Model file for the job. Use its own axes, mm. Face numbers are marked on the shaded views. A direction names the side the tool comes from. Round coordinates to 2 decimals unless told otherwise and drop trailing zeros. Order: outer loops, then holes, each group sorted by start corner. A loop starts at its lowest first (then second) coordinate and runs counter-clockwise, first axis right, second up. Notation, with made-up numbers: (68.25, 38.25) - (94.25, 38.25) arc R27 ccw to (94.25, 63.25) - close; hole circle Ø10 at (65, -9.5). An arc over 180 degrees is marked (long way). Use one line per item in the form item = value.
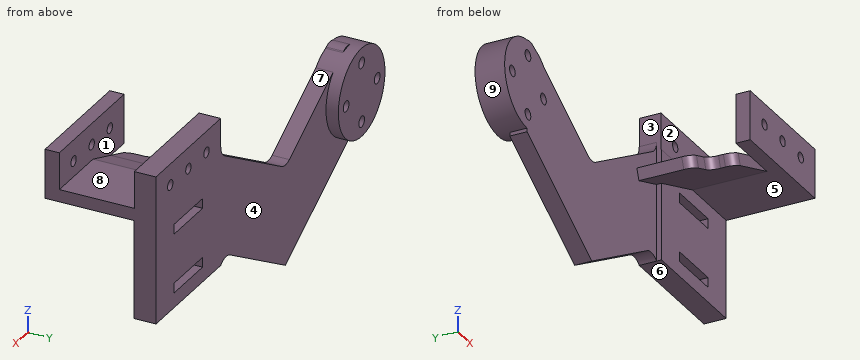
from build123d import *

# Parameters (mm, degrees)
SKETCH_1_W               = 25
SKETCH_1_H               = 10
EXTRUDE_1_DEPTH          = 22.5
SKETCH_2_W               = 25
SKETCH_2_H               = 15.2
CUT_EXTRUDE_1_DEPTH      = 7.5
CUT_EXTRUDE_2_DEPTH      = 36.089172119
CUT_EXTRUDE_2_DEPTH_BACK = 36.089172119
SKETCH_4_R               = 1.03
SKETCH_5_W               = 25
SKETCH_5_H               = 4.5
EXTRUDE_2_DEPTH          = 20
SKETCH_6_W               = 11
SKETCH_6_H               = 2
CUT_EXTRUDE_3_DEPTH      = 4.5
EXTRUDE_3_DEPTH          = 3.5
SKETCH_16_R              = 9
EXTRUDE_4_DEPTH          = 6
CUT_EXTRUDE_4_REACH      = 71.426
SKETCH_17_R              = 1.1
CUT_EXTRUDE_5_REACH      = 73.302
SKETCH_19_W              = 12
SKETCH_19_H              = 15.1
FILLET_7_R               = 3
EXTRUDE_6_REACH          = 72.338
CUT_EXTRUDE_6_REACH      = 72.847
SKETCH_22_W              = 7
SKETCH_22_H              = 5
FILLET_8_R               = 2


with BuildPart() as part:
    # 草图1 → 凸台-拉伸1 (new body)
    with BuildSketch(Plane(origin=(0, 0, 0), x_dir=(1, 0, 0), z_dir=(0, 1, 0))):
        with Locations((12.5, -5)):
            Rectangle(SKETCH_1_W, SKETCH_1_H)
    extrude(amount=EXTRUDE_1_DEPTH)

    # 草图2 → 切除-拉伸1 (cut)
    with BuildSketch(Plane.XY.offset(10)):
        with Locations((12.5, 10.5)):
            Rectangle(SKETCH_2_W, SKETCH_2_H)
    extrude(amount=-CUT_EXTRUDE_1_DEPTH, mode=Mode.SUBTRACT)

    # 草图4 → 切除-拉伸2 (cut, two sides: drawn at the far end of the back side and taken through both)
    with BuildSketch(Plane(origin=(0, 22.5, 0), x_dir=(1, 0, 0), z_dir=(0, 1, 0)).offset(-CUT_EXTRUDE_2_DEPTH_BACK)):
        with Locations(Location((12.5, -5.7, 0), (0, 0, 270))):
            Circle(SKETCH_4_R)
        with Locations(Location((19.5, -5.7, 0), (0, 0, 270))):
            Circle(SKETCH_4_R)
        with Locations(Location((5.5, -5.7, 0), (0, 0, 270))):
            Circle(SKETCH_4_R)
    extrude(amount=CUT_EXTRUDE_2_DEPTH + CUT_EXTRUDE_2_DEPTH_BACK, mode=Mode.SUBTRACT)

    # 草图5 → 凸台-拉伸2 (add)
    with BuildSketch(Plane(origin=(0, 0, 0), x_dir=(-1, 0, 0), z_dir=(0, 0, -1))):
        with Locations((-12.5, 20.25)):
            Rectangle(SKETCH_5_W, SKETCH_5_H)
    extrude(amount=EXTRUDE_2_DEPTH)

    # 草图6 → 切除-拉伸3 (cut)
    with BuildSketch(Plane(origin=(0, 22.5, 0), x_dir=(1, 0, 0), z_dir=(0, 1, 0))):
        with Locations((12.5, 16)):
            Rectangle(SKETCH_6_W, SKETCH_6_H)
        with Locations((12.5, 4)):
            Rectangle(SKETCH_6_W, SKETCH_6_H)
    extrude(amount=-CUT_EXTRUDE_3_DEPTH, mode=Mode.SUBTRACT)

    # 草图15 → 凸台-拉伸3 (add)
    with BuildSketch(Plane(origin=(0, 22.5, 0), x_dir=(1, 0, 0), z_dir=(0, 1, 0))):
        Polygon((0, 17.5), (0, -2.5), (-25, 11.93375673), (-50, -2.5), (-50, 17.5), (-24.967235844, 31.914840335), align=None)
    extrude(amount=-EXTRUDE_3_DEPTH)

    # 草图16 → 凸台-拉伸4 (add)
    with BuildSketch(Plane.XZ.offset(-19)):
        with Locations(Location((-49.655444566, -7.782050808, 0), (0, 0, 267.805955804))):
            Circle(SKETCH_16_R)
    extrude(amount=-EXTRUDE_4_DEPTH)

    # 草图17 → 切除-拉伸4 (cut, up to next)
    with BuildSketch(Plane.XZ.offset(-19), mode=Mode.PRIVATE) as cut_extrude_4_sk1:
        with Locations(Location((-55.655444566, -7.782050808, 0), (0, 0, 90))):
            Circle(SKETCH_17_R)
    cut_extrude_4_tool1 = extrude(cut_extrude_4_sk1.sketch, amount=-CUT_EXTRUDE_4_REACH, mode=Mode.PRIVATE) & part.part
    # 草图17 → 切除-拉伸4 (cut, up to next)
    with BuildSketch(Plane.XZ.offset(-19), mode=Mode.PRIVATE) as cut_extrude_4_sk2:
        with Locations(Location((-43.655444566, -7.782050808, 0), (0, 0, 90))):
            Circle(SKETCH_17_R)
    cut_extrude_4_tool2 = extrude(cut_extrude_4_sk2.sketch, amount=-CUT_EXTRUDE_4_REACH, mode=Mode.PRIVATE) & part.part
    # 草图17 → 切除-拉伸4 (cut, up to next)
    with BuildSketch(Plane.XZ.offset(-19), mode=Mode.PRIVATE) as cut_extrude_4_sk3:
        with Locations(Location((-49.655444566, -1.782050808, 0), (0, 0, 90))):
            Circle(SKETCH_17_R)
    cut_extrude_4_tool3 = extrude(cut_extrude_4_sk3.sketch, amount=-CUT_EXTRUDE_4_REACH, mode=Mode.PRIVATE) & part.part
    # 草图17 → 切除-拉伸4 (cut, up to next)
    with BuildSketch(Plane.XZ.offset(-19), mode=Mode.PRIVATE) as cut_extrude_4_sk4:
        with Locations(Location((-49.655444566, -13.782050808, 0), (0, 0, 90))):
            Circle(SKETCH_17_R)
    cut_extrude_4_tool4 = extrude(cut_extrude_4_sk4.sketch, amount=-CUT_EXTRUDE_4_REACH, mode=Mode.PRIVATE) & part.part
    add(cut_extrude_4_tool1.solids().sort_by_distance((-55.655445, 19, -7.782051))[0], mode=Mode.SUBTRACT)
    add(cut_extrude_4_tool2.solids().sort_by_distance((-43.655445, 19, -7.782051))[0], mode=Mode.SUBTRACT)
    add(cut_extrude_4_tool3.solids().sort_by_distance((-49.655445, 19, -1.782051))[0], mode=Mode.SUBTRACT)
    add(cut_extrude_4_tool4.solids().sort_by_distance((-49.655445, 19, -13.782051))[0], mode=Mode.SUBTRACT)

    # 草图19 → 切除-拉伸5 (cut, up to next)
    with BuildSketch(Plane(origin=(0, 0, 0), x_dir=(-1, 0, 0), z_dir=(0, 0, -1)), mode=Mode.PRIVATE) as cut_extrude_5_sk1:
        with Locations((-6, 10.45)):
            Rectangle(SKETCH_19_W, SKETCH_19_H)
    cut_extrude_5_tool1 = extrude(cut_extrude_5_sk1.sketch, amount=-CUT_EXTRUDE_5_REACH, mode=Mode.PRIVATE) & part.part
    add(cut_extrude_5_tool1.solids().sort_by_distance((6, 10.45, 0))[0], mode=Mode.SUBTRACT)

    # 圆角7
    # the kernel refuses this fillet: 3 mm, written as the material it adds along each edge
    with BuildSketch(Plane(origin=(0, 22.5, -17.5), x_dir=(-0.866025403784437, 0, -0.5000000000000027), z_dir=(0, -1, 0))) as fillet_7_piece_1:
        with BuildLine():
            CenterArc((4.131472029, 3), FILLET_7_R, 196.159495152, 73.840504848)
            Line((1.25, 2.165063509), (0, 0))
            Line((0, 0), (4.131472029, 0))
        make_face()
    extrude(amount=3.5)
    with BuildSketch(Plane(origin=(0, 22.5, 2.5), x_dir=(-0.8660254037844379, 0, -0.5000000000000012), z_dir=(0, -1, 0))) as fillet_7_piece_2:
        with BuildLine():
            CenterArc((FILLET_7_R * 0.57735026919, -FILLET_7_R), FILLET_7_R, 90, 60)
            Line((-FILLET_7_R * 0.288675134595, -FILLET_7_R * 0.5), (0, 0))
            Line((0, 0), (FILLET_7_R * 0.57735026919, 0))
        make_face()
    extrude(amount=3.5)
    with BuildSketch(Plane(origin=(-25, 22.5, -11.93375673), x_dir=(0.8660254037844384, 0, 0.5000000000000003), z_dir=(0, -1, 0))) as fillet_7_piece_3:
        with BuildLine():
            CenterArc((FILLET_7_R * 0.57735026919, FILLET_7_R), FILLET_7_R, 210, 60)
            Line((-FILLET_7_R * 0.288675134595, FILLET_7_R * 0.5), (0, 0))
            Line((0, 0), (FILLET_7_R * 0.57735026919, 0))
        make_face()
    extrude(amount=3.5)
    # the kernel refuses this fillet: 3 mm, written as the material it takes off along each edge
    with BuildSketch(Plane(origin=(-50, 29.947415965, 2.5), x_dir=(0, 0, -1), z_dir=(0, -1, 0))) as fillet_7_2_piece_1:
        with BuildLine():
            CenterArc((4.087559404, 1.079860567), FILLET_7_R, 150, 51.097341704)
            Line((1.489483193, 2.579860567), (0, 0))
            Line((0, 0), (1.288648696, 0))
        make_face()
    extrude(amount=18.394831929, mode=Mode.SUBTRACT)

    # 凸台-拉伸6: up to this face of the body (flat: up to its plane)
    extrude_6_end = Plane(part.part.faces().sort_by_distance((-27.69980279, 19, -14.058564272))[0])
    # 草图21 → 凸台-拉伸6 (add, up to the picked face)
    with BuildSketch(Plane(origin=(0, 2.9, 0), x_dir=(1, 0, 0), z_dir=(0, 1, 0)), mode=Mode.PRIVATE) as extrude_6_sk1:
        Polygon((5.131306451, 0), (12, 0), (-6.793852416, 6.840402867), (-7.597336928, 4.632847313), align=None)
    extrude_6_tool1 = split(extrude(extrude_6_sk1.sketch, amount=EXTRUDE_6_REACH, mode=Mode.PRIVATE), bisect_by=extrude_6_end, keep=Keep.BOTH, mode=Mode.PRIVATE)
    # 草图21 → 凸台-拉伸6 (add, up to the picked face)
    with BuildSketch(Plane(origin=(0, 2.9, 0), x_dir=(1, 0, 0), z_dir=(0, 1, 0)), mode=Mode.PRIVATE) as extrude_6_sk2:
        Polygon((5.131306451, 0), (12, -2.5), (12, 0), align=None)
    extrude_6_tool2 = split(extrude(extrude_6_sk2.sketch, amount=EXTRUDE_6_REACH, mode=Mode.PRIVATE), bisect_by=extrude_6_end, keep=Keep.BOTH, mode=Mode.PRIVATE)
    add(extrude_6_tool1.solids().sort_by(Axis((0.808046, 2.9, -2.903709), (0, 1, 0)))[0])
    add(extrude_6_tool2.solids().sort_by(Axis((9.710435, 2.9, 0.833333), (0, 1, 0)))[0])

    # 草图22 → 切除-拉伸6 (cut, up to next)
    with BuildSketch(Plane(origin=(1.403733341, 0, -3.856725658), x_dir=(-0.9396926207859082, 0, -0.3420201433256691), z_dir=(0.3420201433256691, 0, -0.9396926207859082)), mode=Mode.PRIVATE) as cut_extrude_6_sk1:
        with Locations((5.223688551, 5.4)):
            Rectangle(SKETCH_22_W, SKETCH_22_H)
    cut_extrude_6_tool1 = extrude(cut_extrude_6_sk1.sketch, amount=-CUT_EXTRUDE_6_REACH, mode=Mode.PRIVATE) & part.part
    add(cut_extrude_6_tool1.solids().sort_by_distance((-3.504928, 5.4, -5.643332))[0], mode=Mode.SUBTRACT)

    # 圆角8
    fillet_8_edges = [part.edges().sort_by_distance(p)[0] for p in [
        (-7.195594672, 7.9, -5.73662509),
        (-0.617746326, 2.9, -3.342484086),
        (-0.617746326, 7.9, -3.342484086),
    ]]
    fillet(fillet_8_edges, radius=FILLET_8_R)


solid = part.part
(1) Slice it at C-C on x = 2.5. Give the cut face in (y, z).
Report:
outline = (0, 0) - (2.9, 0) - (2.9, 10) - (0, 10) - close; (2.9, -3.46) - (18, -3.46) - (18, -20) - (22.5, -20) - (22.5, 10) - (18.1, 10) - (18.1, 2.5) - (18, 2.5) - (18, -0.96) - (2.9, -0.96) - close
(2) Tool access for the marked faces 5, 6, 7, 8 and 9: list every direction of +Z, -Z, +X, -X, +Y, -Y with a clear straight run to the whole face (end or side of a thin tool).
Report:
face_5 = -Z, +X, -Y
face_6 = -Z, +X, +Y, -Y
face_7 = +Z, +Y, -Y
face_8 = +Z, +X, -X
face_9 = +Y
(3) Slice it at D-D on y = 21.25. Count the separate pieces of the cut face and the enclosed holes in it, then the cut area to 3 significant figures.
Report:
separate_pieces = 1
enclosed_holes = 9
area = 1,800 mm2
(4) Pull direction Y, two halves, no side cores. Call the marked faces 1, 2, 3 and 4: released by +Y, released by -Y, zero draft, split by the parting line, or undercut.
Report:
face_1 = undercut
face_2 = undercut
face_3 = zero draft
face_4 = released by +Y
(5) Slice it at B-B on y = 16.75. Give the cut face in (x, z), then the cut area to 3 significant figures.
Report:
outline = (-7.6, -4.63) - (-6.79, -6.84) - (12, 0) - (25, 0) - (25, 2.5) - (12, 2.5) - close
area = 80.5 mm2
(6) Pin check, flat tips, straight feed: pin 1 (2.5 mm diameter, centred on x = -3.5, z = -4.5, fed in from -Y); pin 2 (12 mm diameter, centred on y = 22, z = 4, fed in from -X); pin 3 (5 mm diameter, centred on x = -19, z = -9, fed in from -Y). Stop position of each tip, or through.
Report:
pin_1 = 7.89
pin_2 = -56.55
pin_3 = 19
(7) Probe probe 1 along X at (y, z) = (0.65, 5.7); probe 2 along Z at (x, y) = (12.5, 20.25); probe 3 along Z at (x, y) = (15.5, 20.25). List the from-to ranges inside material, lowest first. Write a range as [from, to].
Report:
probe_1 = [0, 4.47], [6.53, 11.47], [13.53, 18.47], [20.53, 25]
probe_2 = [-20, -17], [-15, -5], [-3, 4.67], [6.73, 10]
probe_3 = [-20, -17], [-15, -5], [-3, 10]
(8) Slice it at A-A on x = 15. Give the cut face in (y, z).
Report:
outline = (0, 0) - (18, 0) - (18, -3) - (22.5, -3) - (22.5, 10) - (18.1, 10) - (18.1, 2.5) - (2.9, 2.5) - (2.9, 10) - (0, 10) - close; (18, -20) - (22.5, -20) - (22.5, -17) - (18, -17) - close; (18, -15) - (22.5, -15) - (22.5, -5) - (18, -5) - close
